from build123d import *

# Parameters (mm, degrees)
SKETCH1_W           = 7.3
SKETCH1_H           = 14.9
SKETCH1_W_2         = 4.7
SKETCH1_H_2         = 12.3
BOSS_EXTRUDE1_DEPTH = 16
BOSS_EXTRUDE2_START = 12
SKETCH4_W           = 4.7
SKETCH4_H           = 2.15
BOSS_EXTRUDE2_DEPTH = 4
SKETCH5_R           = 1
CUT_EXTRUDE1_DEPTH  = 15


with BuildPart() as part:
    # Sketch1 → Boss-Extrude1 (new body)
    with BuildSketch(Plane.XY):
        with Locations((2.35, 6.15)):
            Rectangle(SKETCH1_W, SKETCH1_H)
        with Locations((2.35, 6.15)):
            Rectangle(SKETCH1_W_2, SKETCH1_H_2, mode=Mode.SUBTRACT)
    extrude(amount=BOSS_EXTRUDE1_DEPTH)

    # Sketch4 → Boss-Extrude2 (add)
    with BuildSketch(Plane.XY.offset(BOSS_EXTRUDE2_START)):
        with Locations((2.35, 1.075)):
            Rectangle(SKETCH4_W, SKETCH4_H)
        with Locations((2.35, 11.225)):
            Rectangle(SKETCH4_W, SKETCH4_H)
    extrude(amount=BOSS_EXTRUDE2_DEPTH)

    # Sketch5 → Cut-Extrude1 (cut)
    with BuildSketch(Plane.ZY.offset(1.3)):
        with Locations((8.8, 6.4)):
            Circle(SKETCH5_R)
    extrude(amount=-CUT_EXTRUDE1_DEPTH, mode=Mode.SUBTRACT)


solid = part.part
The model under review builds one solid part; all positions refer to its coordinate system, in mm. A direction names the side the tool comes from. Round coordinates to 2 decimals unless told otherwise and drop trailing zeros. Loops run counter-clockwise (first coordinate to the right, second up) from the corner with the lowest first, then second, coordinate; pieces in that order, holes last. Notation, with made-up numbers: M 59.25,-16.75 L 108.25,-16.75 A20 cw 108.25,-4.75 Z; hole C 5.5,41 d2. An arc over 180 degrees is marked long. Answer as a JSON object with one key per item and string values.
Item 1: For line 1 along Y through (x, z) = (0.5, 10); line 2 along X through (y, z) = (10.5, 9.5); line 3 along Y through (x, z) = (5, 8.8), list the stretches that pass through material, from the lowest coordinate up.
Check sheet entries:
{"line 1": "-1.3 to 0, 12.3 to 13.6", "line 2": "-1.3 to 0, 4.7 to 6", "line 3": "-1.3 to 5.4, 7.4 to 13.6"}
Item 2: We need section C-C, the plane z = 8.8. State the section outline as (x, y) points, and give its area (3 significant figures).
Check sheet entries:
{"outline": "M -1.3,-1.3 L 6,-1.3 L 6,5.4 L 4.7,5.4 L 4.7,0 L 0,0 L 0,5.4 L -1.3,5.4 Z; M -1.3,7.4 L 0,7.4 L 0,12.3 L 4.7,12.3 L 4.7,7.4 L 6,7.4 L 6,13.6 L -1.3,13.6 Z", "area": "45.8 mm2"}
Item 3: We need section D-D, the plane x = 0.25. State the section outline as (y, z) points, and give its area (3 significant figures).
Check sheet entries:
{"outline": "M -1.3,0 L 0,0 L 0,12 L 2.15,12 L 2.15,16 L -1.3,16 Z; M 10.15,12 L 12.3,12 L 12.3,0 L 13.6,0 L 13.6,16 L 10.15,16 Z", "area": "58.8 mm2"}
Item 4: The part is to be moulded in two halves that separate along Y. For faces 4 (the face through (2, 1, 12)), 5 (the face through (2, 13.6, 8)), 6 (the face through (5, 6, 0)), 7 (the face through (2, 0, 6)), say which applies: +Y half, -Y half, draft (parallel to the pull), parting line (faces both ways), or undercut.
Check sheet entries:
{"face 4": "undercut", "face 5": "+Y half", "face 6": "draft", "face 7": "undercut"}
Item 5: Tool access review of faces 1 (the face through (2, 2.15, 14)), 2 (the face through (2, 11, 12)), 3 (the face through (6, 4, 8)): name each direction out of +Z, -Z, +X, -X, +Y, -Y from which nothing blocks a thin tool from reaching the whole face with its end or side.
Check sheet entries:
{"face 1": "+Z, -Z", "face 2": "-Z", "face 3": "+Z, -Z, +X, +Y, -Y"}
Item 6: Clearance check with a flat-ended pin moving along its axis: P1, Ø0.6, axis at x = 2.5, y = 11, coming from the -Z side. State where the tip first meets the part, or that it passes through.
Check sheet entries:
{"P1": "z = 12"}
Item 7: We need section A-A, the plane y = 6.4. State the section outline as (x, z) points, and give its area (3 significant figures).
Check sheet entries:
{"outline": "M -1.3,0 L 0,0 L 0,7.8 L -1.3,7.8 Z; M -1.3,9.8 L 0,9.8 L 0,16 L -1.3,16 Z; M 4.7,0 L 6,0 L 6,7.8 L 4.7,7.8 Z; M 4.7,9.8 L 6,9.8 L 6,16 L 4.7,16 Z", "area": "36.4 mm2"}
Item 8: We need section B-B, the plane z = 1. State the section outline as (x, y) points, and give its area (3 significant figures).
Check sheet entries:
{"outline": "M -1.3,-1.3 L 6,-1.3 L 6,13.6 L -1.3,13.6 Z; hole M 0,0 L 4.7,0 L 4.7,12.3 L 0,12.3 Z", "area": "51.0 mm2"}
